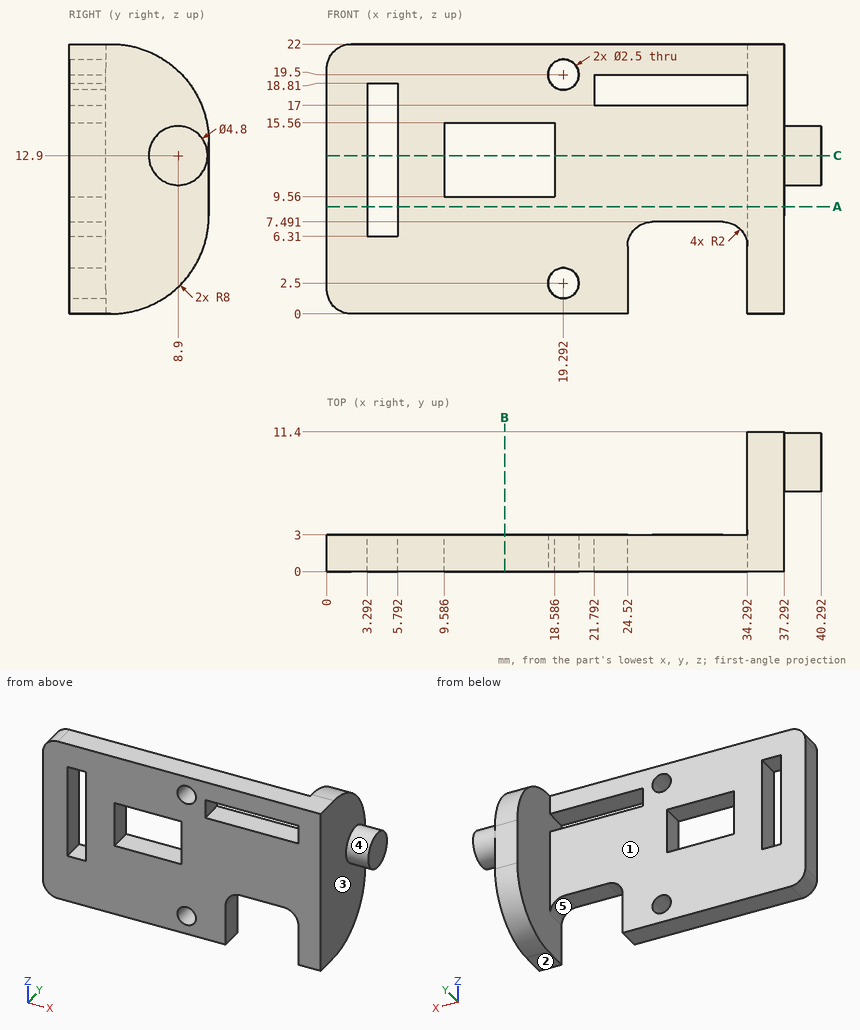
Study the drawing (mm; zero at the part's minimum x, y, z) and answer. A direction names the side the tool comes from. Give positions to 0.01 mm unless a question says otherwise; leave off trailing zeros. Write each loop counter-clockwise with the first axis right and the second up, starting at its lowest first coordinate (ties: lowest second). Pieces come first, ordered by that corner, then holes. Notation, with made-up numbers: (14.25, -36) - (35.25, -36) arc R15 cw to (35.25, -23) - close; hole circle Ø4 at (-26, 57). An arc over 180 degrees is marked (long way). Write item = value, one per line. Start each with the question number.
Item 1: Find section A-A (z = 8.75). Give the vertices of the cut face in (x, y).
Item 2: A tool of negligible diameter and unlimited length cuts with its end or side. For the marked faces 1 and 2, from which of +Z, -Z, +X, -X, +Y, -Y can it reach the whole face along a straight path? Write none if from no direction.
Item 3: Find section C-C (z = 12.9). State how many separate pieces and enclosed holes the cut face has, then the cut area to 3 significant figures.
Item 4: Find the intervals of material crossed by probe 1 along X at (y, z) = (2.25, 15) (1 decimal); probe 2 along X at (y, z) = (1.4, 2.5); probe 3 along X at (y, z) = (1.75, 4.5), in increasing order. Write a range as [from, to].
Item 5: Each of these flat-tipped pins is pushed along its axis until it touches: P1, Ø3.5, axis at y = 5, z = 16, coming from the +X side; P2, Ø2.5, axis at x = 30.5, y = 1, coming from the -Z side; P3, Ø5, axis at x = 24, z = 17, coming from the +Y side; P4, Ø2, axis at x = 19.5, y = 4.5, coming from the +Z side. Where does it stop, or does it pass through?
Item 6: The mould has two halves that part along X. Classify the marked faces 3, 4 and 5: +X half, -X half, draft (parallel to the pull), parting line (faces both ways), or undercut.
Item 7: Find section B-B (x = 14.5). Give the vertices of the cut face in (y, z).
Response:
q1.outline = (0, 0) - (3.29, 0) - (3.29, 3) - (0, 3) - close; (5.79, 0) - (37.29, 0) - (37.29, 11.4) - (34.29, 11.4) - (34.29, 3) - (5.79, 3) - close
q2.face_1 = +Z, -Z, -X, +Y
q2.face_2 = -Z, +X, -X, +Y, -Y
q3.separate_pieces = 3
q3.enclosed_holes = 0
q3.area = 117 mm²
q4.probe_1 = [0, 3.3], [5.8, 9.6], [18.6, 37.3]
q4.probe_2 = [0, 18.04], [20.54, 24.52], [34.29, 37.29]
q4.probe_3 = [0, 24.52], [34.29, 37.29]
q5.P1 = 37.29
q5.P2 = 7.49
q5.P3 = 3
q5.P4 = through
q6.face_3 = +X half
q6.face_4 = draft
q6.face_5 = undercut
q7.outline = (0, 0) - (3, 0) - (3, 9.56) - (0, 9.56) - close; (0, 15.56) - (3, 15.56) - (3, 22) - (0, 22) - close
